```python
from build123d import *

# Parameters (mm, degrees)
SKETCH1_W           = 39.5
SKETCH1_H           = 20
BOSS_EXTRUDE1_DEPTH = 28
BOSS_EXTRUDE2_DEPTH = 6.5
SKETCH3_W           = 39.5
SKETCH3_H           = 20
BOSS_EXTRUDE3_DEPTH = 9.5
SKETCH4_R           = 4
BOSS_EXTRUDE4_DEPTH = 6
SKETCH5_W           = 7
SKETCH5_H           = 4
BOSS_EXTRUDE5_DEPTH = 8


with BuildPart() as part:
    # Sketch1 → Boss-Extrude1 (new body)
    with BuildSketch(Plane(origin=(0, 0, 0), x_dir=(1, 0, 0), z_dir=(0, 1, 0))):
        with Locations((-23.401244555, 9.028670505)):
            Rectangle(SKETCH1_W, SKETCH1_H)
    extrude(amount=BOSS_EXTRUDE1_DEPTH)

    # Sketch2 → Boss-Extrude2 (add)
    with BuildSketch(Plane(origin=(0, 28, 0), x_dir=(1, 0, 0), z_dir=(0, 1, 0))):
        Polygon((-43.151244555, 19.028670505), (-51.668180021, 19.028670505), (-51.668180021, -0.971329495), (-43.151244555, -0.971329495), (-3.651244555, -0.971329495), (4.86569091, -0.971329495), (4.86569091, 19.028670505), (-3.651244555, 19.028670505), align=None)
    extrude(amount=BOSS_EXTRUDE2_DEPTH)

    # Sketch3 → Boss-Extrude3 (add)
    with BuildSketch(Plane(origin=(0, 34.5, 0), x_dir=(1, 0, 0), z_dir=(0, 1, 0))):
        with Locations((-23.401244555, 9.028670505)):
            Rectangle(SKETCH3_W, SKETCH3_H)
    extrude(amount=BOSS_EXTRUDE3_DEPTH)

    # Sketch4 → Boss-Extrude4 (add)
    with BuildSketch(Plane(origin=(0, 44, 0), x_dir=(1, 0, 0), z_dir=(0, 1, 0))):
        with Locations(Location((-12.651244555, 9.028670505, 0), (0, 0, 90))):
            Circle(SKETCH4_R)
    extrude(amount=BOSS_EXTRUDE4_DEPTH)

    # Sketch5 → Boss-Extrude5 (add)
    with BuildSketch(Plane(origin=(-3.651244555, 0, 0), x_dir=(0, 0, -1), z_dir=(1, 0, 0))):
        with Locations((9.028670505, 4)):
            Rectangle(SKETCH5_W, SKETCH5_H)
    extrude(amount=BOSS_EXTRUDE5_DEPTH)


solid = part.part
```
Source: CAD feature listing. Evaluate the final solid. Frame: model axes, mm. A direction names the side the tool comes from. Give positions to 0.01 mm unless a question says otherwise; leave off trailing zeros. Loops run counter-clockwise (first coordinate to the right, second up) from the corner with the lowest first, then second, coordinate; pieces in that order, holes last. Notation, with made-up numbers: (17, 43) -> (43, 43) arc R27 cw to (43, 59) -> close; hole circle Ø3 at (-37, 21.25). An arc over 180 degrees is marked (long way). Use a Markdown table: item, result. Add a question column.
(1) First-contact query: pin 1 Ø7 at (x, z) = (-49, -5.5) entering from +Y; pin 2 Ø2 at (y, z) = (7.5, -2) entering from +X; pin 3 Ø1 at (x, z) = (-38, -3) entering from +Y. Flat tips, straight axial feed; report the tip coordinate or a pass-through.
(2) Section query D-D (y = 37). Output: boundary loops of the cut face in (x, z), then the cut area to 3 significant figures.
(3) Access query for faces 4 (the face through (1, 28, -9)), 5 (the face through (-3.651, 39, -9)), 6 (the face through (4.349, 4, -9)), 7 (the face through (-43.151, 39, -9)). Directions: +Z, -Z, +X, -X, +Y, -Y. A direction counts if a zero-diameter tool reaches every point of the face in a straight line with its end or side. Return the directions, or none.
(4) Ray query, line 1 (Y direction, x = -16.5, z = -3.75); line 2 (X direction, y = 2, z = -16.25); line 3 (X direction, y = 3.5, z = -11.5). Return the intervals inside material, ascending.
(5) Section query B-B (z = -15.75). Output: boundary loops of the cut face in (x, y), then the cut area to 3 significant figures.
(6) Pull-direction query (Y, two-part tool) for faces 1 (the face through (-43.151, 14, -9)), 2 (the face through (0, 6, -9)), 3 (the face through (-24, 44, -9)); classes: +Y half, -Y half, draft (parallel to the pull), parting line (faces both ways), or undercut.
(7) Section query A-A (x = -1). Output: boundary loops of the cut face in (y, z), then the cut area to 3 significant figures.
(8) Section query C-C (x = -31). Output: boundary loops of the cut face in (y, z).
Checked values:
| question | item | result |
|---|---|---|
| 1 | pin 1 | y = 34.5 |
| 1 | pin 2 | x = -3.65 |
| 1 | pin 3 | y = 44 |
| 2 | outline | (-43.15, -19.03) -> (-3.65, -19.03) -> (-3.65, 0.97) -> (-43.15, 0.97) -> close |
| 2 | area | 790 mm^2 |
| 3 | face 4 | +Z, -Z, +X |
| 3 | face 5 | +Z, -Z, +X, +Y |
| 3 | face 6 | +Z, -Z, +X, -Y |
| 3 | face 7 | +Z, -Z, -X, +Y |
| 4 | line 1 | 0 to 44 |
| 4 | line 2 | -43.15 to -3.65 |
| 4 | line 3 | -43.15 to 4.35 |
| 5 | outline | (-51.67, 28) -> (-43.15, 28) -> (-43.15, 0) -> (-3.65, 0) -> (-3.65, 28) -> (4.87, 28) -> (4.87, 34.5) -> (-3.65, 34.5) -> (-3.65, 44) -> (-43.15, 44) -> (-43.15, 34.5) -> (-51.67, 34.5) -> close |
| 5 | area | 1,850 mm^2 |
| 6 | face 1 | draft |
| 6 | face 2 | undercut |
| 6 | face 3 | +Y half |
| 7 | outline | (2, -12.53) -> (6, -12.53) -> (6, -5.53) -> (2, -5.53) -> close; (28, -19.03) -> (34.5, -19.03) -> (34.5, 0.97) -> (28, 0.97) -> close |
| 7 | area | 158 mm^2 |
| 8 | outline | (0, -19.03) -> (44, -19.03) -> (44, 0.97) -> (0, 0.97) -> close |
